Job drawing, mm, ordinate dimensions from the low corner. One solid piece. A direction names the side the tool comes from. Coordinates: 2 decimals unless noted, no trailing zeros. Order: outer loops, then holes, each group sorted by start corner. A loop starts at its lowest first (then second) coordinate and runs counter-clockwise, first axis right, second up. Notation, with made-up numbers: (58.5, -25.75) - (85.5, -25.75) arc R11 ccw to (85.5, -15.75) - close; hole circle Ø10 at (42, 60.25). An arc over 180 degrees is marked (long way). Use a Markdown table: item, result. Add a question column.
1) Wall check: L1, parallel to Y at x = 79, z = 22; L2, parallel to Z at x = 144.5, y = 43.5; L3, parallel to Y at x = 59, z = 55. Give the ranges that are in metal, low to high. Write a range as [from, to].
2) Saw through at C-C on y = 80. List the corners of the cut face in (x, z), then the cut area to 3 significant figures.
3) Saw through at A-A on z = 90.5. List the corners of the cut face in (x, y), then the cut area to 3 significant figures.
4) Saw through at B-B on x = 16.5. List the corners of the cut face in (y, z).
5) Drop flat-ended pins along their axis: P1, Ø6, axis at y = 60, z = 70, coming from the -X side; P2, Ø1.5, axis at x = 132.5, y = 78, coming from the +Z side; P3, Ø15, axis at x = 72.5, y = 38, coming from the +Z side; P4, Ø6, axis at x = 135, z = 29.5, coming from the -Y side. Give the stop position or say it passes through.
6) Saw through at D-D on x = 181. List the corners of the cut face in (y, z), then the cut area to 3 significant figures.
7) Two-plate mould, pull along X, no slides. Class the marked faces 4, 5 and 6: +X half, -X half, draft (parallel to the pull), parting line (faces both ways), or undercut.
8) Tool access for the marked faces 1, 2 and 3: list every direction of +Z, -Z, +X, -X, +Y, -Y with a clear straight run to the whole face (end or side of a thin tool).
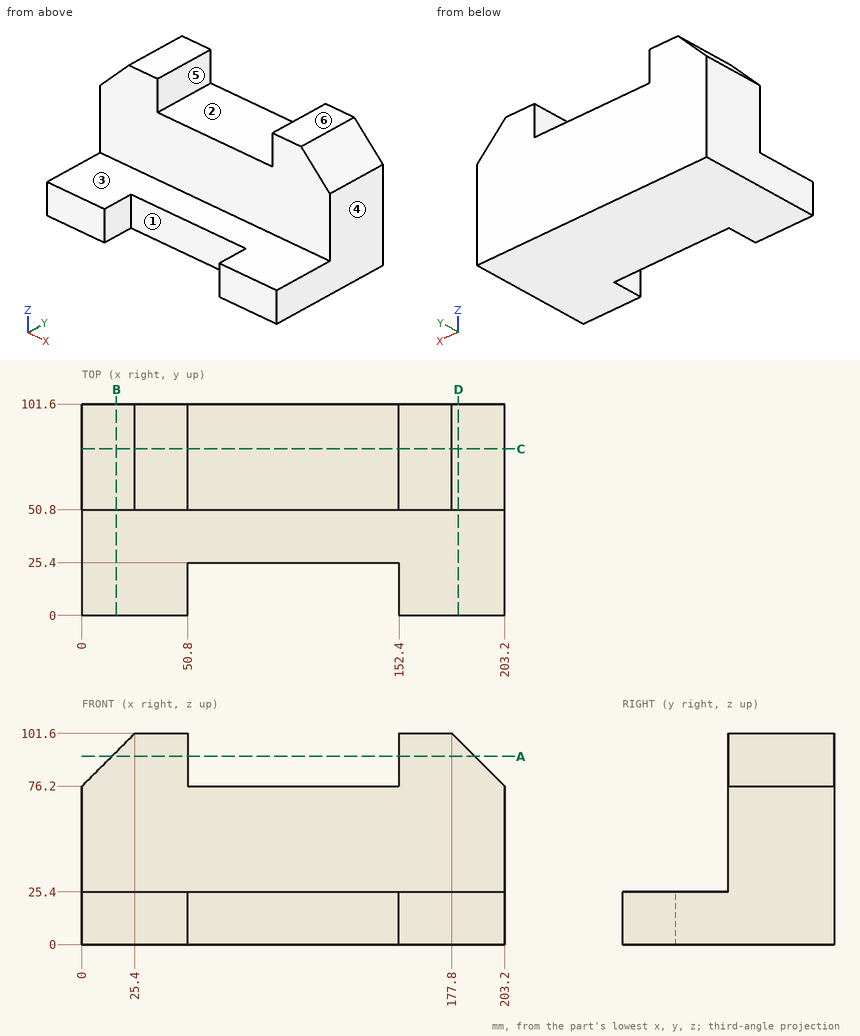
Results are:
| question | item | result |
|---|---|---|
| 1 | L1 | [25.4, 101.6] |
| 1 | L2 | [0, 25.4] |
| 1 | L3 | [50.8, 101.6] |
| 2 | outline | (0, 0) - (203.2, 0) - (203.2, 76.2) - (177.8, 101.6) - (152.4, 101.6) - (152.4, 76.2) - (50.8, 76.2) - (50.8, 101.6) - (25.4, 101.6) - (0, 76.2) - close |
| 2 | area | 17,400 mm2 |
| 3 | outline | (14.3, 50.8) - (50.8, 50.8) - (50.8, 101.6) - (14.3, 101.6) - close; (152.4, 50.8) - (188.9, 50.8) - (188.9, 101.6) - (152.4, 101.6) - close |
| 3 | area | 3,710 mm2 |
| 4 | outline | (0, 0) - (101.6, 0) - (101.6, 92.7) - (50.8, 92.7) - (50.8, 25.4) - (0, 25.4) - close |
| 5 | P1 | x = 0 |
| 5 | P2 | z = 76.2 |
| 5 | P3 | z = 25.4 |
| 5 | P4 | y = 50.8 |
| 6 | outline | (0, 0) - (101.6, 0) - (101.6, 98.4) - (50.8, 98.4) - (50.8, 25.4) - (0, 25.4) - close |
| 6 | area | 6,290 mm2 |
| 7 | face 4 | +X half |
| 7 | face 5 | undercut |
| 7 | face 6 | draft |
| 8 | face 1 | +Z, -Z, -Y |
| 8 | face 2 | +Z, +Y, -Y |
| 8 | face 3 | +Z, +X, -X, -Y |
